Verification items for the finished model (mm, model axes). Face numbers are marked on the shaded views. Round coordinates to 2 decimals unless told otherwise and drop trailing zeros. Loops run counter-clockwise (first coordinate to the right, second up) from the corner with the lowest first, then second, coordinate; pieces in that order, holes last.
from build123d import *

# Parameters (mm, degrees)
BOSS_EXTRUDE1_DEPTH     = 36
FILLET1_R               = 6
SKETCH2_R               = 2.05
CUT_EXTRUDE1_DEPTH      = 39.157568057
LPATTERN1_COUNT         = 2
LPATTERN1_PITCH         = 8
MIRROR1_COPY_1_SKETCH_R = 2.05
MIRROR1_COPY_1_DEPTH    = 39.157568057


with BuildPart() as part:
    # Sketch1 → Boss-Extrude1 (new body)
    with BuildSketch(Plane.XY):
        Polygon((0, 0), (4, 0), (4, 2), (3, 2), (3, 10), (4, 10), (4, 12), (0, 12), align=None)
    extrude(amount=-BOSS_EXTRUDE1_DEPTH)

    # Fillet1
    fillet1_edges = [part.edges().sort_by_distance(p)[0] for p in [
        (2, 12, 0),
        (2, 0, 0),
        (2, 0, -36),
        (2, 12, -36),
    ]]
    fillet(fillet1_edges, radius=FILLET1_R - 0.0001)  # a hair under: the kernel refuses the full size

    # Sketch2 → Cut-Extrude1 (cut, through all)
    with BuildSketch(Plane.ZY):
        with Locations(Location((-30, 6, 0), (0, 0, 270))):
            Circle(SKETCH2_R)
    cut_extrude1 = extrude(amount=-CUT_EXTRUDE1_DEPTH, mode=Mode.SUBTRACT)

    # LPattern1: Cut-Extrude1 ×2
    with Locations(*[(0, 0, i * LPATTERN1_PITCH) for i in range(1, LPATTERN1_COUNT)]):
        add(cut_extrude1, mode=Mode.SUBTRACT)

    # Mirror1: Cut-Extrude1 across plane
    add(cut_extrude1.mirror(Plane.XY.offset(-18)), mode=Mode.SUBTRACT)

    # Mirror1 copy 1 sketch → Mirror1 copy 1 (cut, through all)
    with BuildSketch(Plane(origin=(0, 0, -44), x_dir=(0, 0, -1), z_dir=(-1, 0, 0))):
        with Locations((-30, -6)):
            Circle(MIRROR1_COPY_1_SKETCH_R)
    extrude(amount=-MIRROR1_COPY_1_DEPTH, mode=Mode.SUBTRACT)


solid = part.part
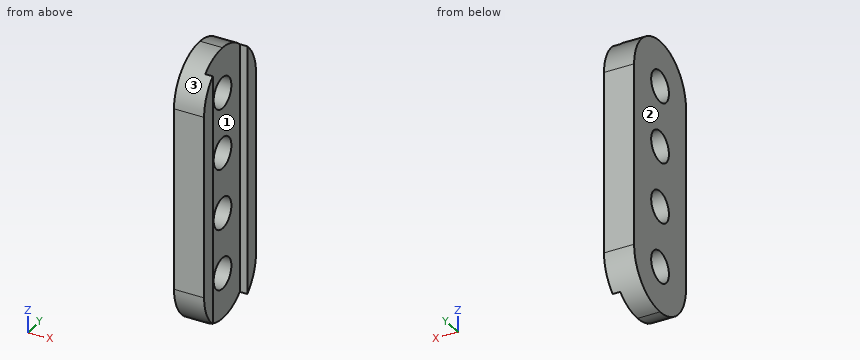
1. Section check C-C (z = -3). Enter the section's corners in (x, y), then the cut area to 3 significant figures.
2. Scan lines: L1, parallel to Z at x = 1.9, y = 6; L2, parallel to Y at x = 2.6, z = -14; L3, parallel to Y at x = 3.6, z = -28.5. Record each from-to range of solid material in increasing order.
3. Section check B-B (x = 1.4). Give the number of separate pieces and of enclosed holes in the cut face, then the cut area to 3 significant figures.
4. Release check for a two-part mould opening along Y. For the marked faces 1, 2 and 3 record: released by +Y, released by -Y, zero draft, split by the parting line, or undercut.
5. Section check A-A (z = -22). Enter the section's corners in (x, y).
6. Section check D-D (z = -12.5). Enter the section's corners in (x, y).
7. Gauge pin test, flat end, axial feed: P1, Ø6.5, axis at y = 6, z = -22, coming from the +X side. Record the tip position at first contact, or that the pin passes through.
Taken from the geometry:
1. outline: (0, 0.8) - (4, 0.8) - (4, 2) - (3, 2) - (3, 10) - (4, 10) - (4, 11.2) - (0, 11.2) - close
1. area: 33.6 mm2
2. L1: z = -36 to -32.05, -27.95 to -24.05, -19.95 to -16.05, -11.95 to -8.05, -3.95 to 0
2. L2: y = 0 to 3.95, 8.05 to 12
2. L3: y = 0 to 2, 10 to 12
3. separate pieces: 1
3. enclosed holes: 4
3. area: 348 mm2
4. face 1: undercut
4. face 2: zero draft
4. face 3: released by -Y
5. outline: (0, 0) - (4, 0) - (4, 2) - (3, 2) - (3, 3.95) - (0, 3.95) - close; (0, 8.05) - (3, 8.05) - (3, 10) - (4, 10) - (4, 12) - (0, 12) - close
6. outline: (0, 0) - (4, 0) - (4, 2) - (3, 2) - (3, 4.6) - (0, 4.6) - close; (0, 7.4) - (3, 7.4) - (3, 10) - (4, 10) - (4, 12) - (0, 12) - close
7. P1: stops at x = 3
